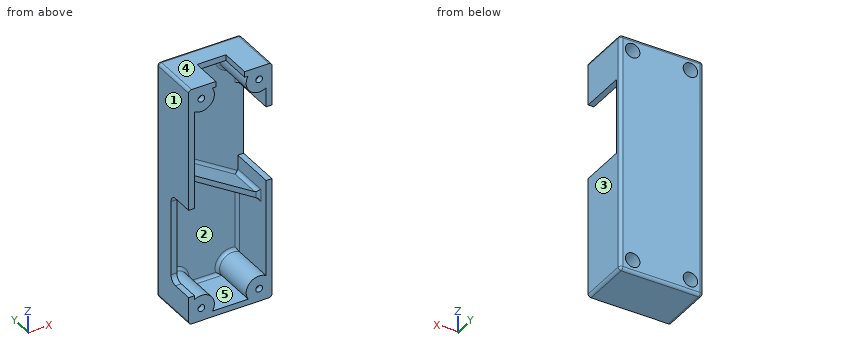
Autodesk Inventor part; units mm, degrees
ref_plane "YZ Plane" through (0, 0, 0) normal (1, 0, 0) x (0, 1, 0)
ref_plane "XZ Plane" through (0, 0, 0) normal (0, 1, 0) x (-1, 0, 0)
ref_plane "XY Plane" through (0, 0, 0) normal (0, 0, 1) x (1, 0, 0)
sketch "Sketch1" plane through (0, 0, 0) normal (0, 1, 0) x (-1, 0, 0)
  line L0 (-4.1759, -63.8889) -> (-35.6719, -63.8889)
  line L1 (-35.6719, -63.8889) -> (-35.6719, 36.1871)
  line L2 (-35.6719, 36.1871) -> (-4.1759, 36.1871)
  line L3 (-4.1759, 36.1871) -> (-4.1759, -63.8889)
  line L4 (-1.6359, -66.4289) -> (-38.2119, -66.4289)
  line L5 (-38.2119, -66.4289) -> (-38.2119, 38.7271)
  line L6 (-38.2119, 38.7271) -> (-1.6359, 38.7271)
  line L7 (-1.6359, 38.7271) -> (-1.6359, -66.4289)
  point P0 (0, 0)
  dimension "d0" = 100.076
  dimension "d1" = 31.496
  dimension "d2" = 2.54
  dimension "d3" = 2.54
  dimension "d4" = 2.54
  dimension "d5" = 2.54
extrude "Extrusion1" add sketch "Sketch1" along normal blind 22.86 contours L0 L1 L2 L3 | L4 L5 L6 L7
extrude "Extrusion2" cut sketch "Sketch1" along normal blind 20.32 contours L0 L1 L2 L3
sketch "Sketch2" plane through (0, 0, 0) normal (0, -1, 0) x (1, 0, 0)
  line L0 (35.6719, 36.1871) -> (35.6719, -63.8889)
  line L1 (38.2119, 38.7271) -> (38.2119, -66.4289)
  line L2 (38.2119, 19.6771) -> (35.6719, 19.6771)
  line L3 (38.2119, -13.3429) -> (35.6719, -13.3429)
  line L4 (4.1759, 36.1871) -> (35.6719, 36.1871)
  point P0 (0, 0)
  point P1 (36.9419, 19.6771)
  point P2 (36.9419, -13.3429)
  dimension "d10" = 16.51
  dimension "d11" = 33.02
extrude "Extrusion3" cut sketch "Sketch2" against normal blind 20.32
sketch "Sketch3" plane through (1.6359, 0, 38.7271) normal (0, 0, 1) x (1, 0, 0)
  line L0 (11.938, 0) -> (24.638, 0)
  line L1 (24.638, 0) -> (24.638, 13.5128)
  line L2 (24.638, 13.5128) -> (11.938, 13.5128)
  line L3 (11.938, 13.5128) -> (11.938, 0)
  line L4 (0, 0) -> (0, 22.86)
  line L5 (36.576, 0) -> (36.576, 22.86)
  line L6 (36.576, 22.86) -> (0, 22.86)
  line L7 (18.288, 22.86) -> (18.288, 0)
  point P0 (-1.6359, 0)
  dimension "d16" = 13.5128
  dimension "d17" = 12.7
  dimension "d18" = 12.7
extrude "Extrusion4" cut sketch "Sketch3" against normal blind 2.54
sketch "Sketch4" plane through (1.6359, 0, -66.4289) normal (-1, 0, 0) x (0, 0, 1)
  line L0 (12.192, 0) -> (51.3334, 0)
  line L1 (51.3334, 0) -> (51.3334, 12.7)
  line L2 (51.3334, 12.7) -> (12.192, 12.7)
  line L3 (12.192, 12.7) -> (12.192, 0)
  line L4 (0, 0) -> (0, 22.86)
  point P0 (66.4289, 0)
  point P1 (31.7627, 0)
  dimension "d21" = 12.192
  dimension "d22" = 12.7
  dimension "d23" = 39.1414
extrude "Extrusion5" cut sketch "Sketch4" against normal blind 2.54
sketch "Sketch5" plane through (0, 22.86, 0) normal (0, 1, 0) x (1, 0, 0)
  circle A0 centre (32.6239, -33.1391) radius 1.4732
  line L0 (38.2119, -38.7271) -> (38.2119, 66.4289)
  line L1 (1.6359, -38.7271) -> (38.2119, -38.7271)
  line L2 (1.6359, 66.4289) -> (1.6359, -38.7271)
  line L3 (1.6359, 13.8509) -> (38.2119, 13.8509)
  line L4 (19.9239, 66.4289) -> (19.9239, -38.7271)
  circle A1 centre (7.2239, -33.1391) radius 1.4732
  circle A2 centre (32.6239, 60.8409) radius 1.4732
  circle A3 centre (7.2239, 60.8409) radius 1.4732
  circle A4 centre (32.6239, -33.1391) radius 3.175
  line L5 (38.2119, -31.941) -> (38.2119, -34.3372)
  line L6 (31.4257, -38.7271) -> (33.822, -38.7271)
  arc A5 (38.2119, -31.941) -> (31.4257, -38.7271) centre (32.6239, -33.1391) ccw
  line L7 (38.2119, -34.3372) -> (38.2119, -38.7271)
  line L8 (38.2119, -38.7271) -> (33.822, -38.7271)
  line L9 (38.2119, -38.7271) -> (1.6359, -38.7271)
  circle A6 centre (7.2239, -33.1391) radius 3.175
  line L10 (1.6359, -31.941) -> (1.6359, -34.3372)
  arc A7 (8.422, -38.7271) -> (1.6359, -31.941) centre (7.2239, -33.1391) ccw
  line L11 (1.6359, -34.3372) -> (1.6359, -38.7271)
  line L12 (38.2119, 66.4289) -> (38.2119, -38.7271)
  line L13 (1.6359, -38.7271) -> (1.6359, 66.4289)
  circle A8 centre (32.6239, 60.8409) radius 3.175
  arc A9 (31.4257, 66.4289) -> (38.2119, 59.6428) centre (32.6239, 60.8409) ccw
  circle A10 centre (7.2239, 60.8409) radius 3.175
  arc A11 (1.6359, 59.6428) -> (8.422, 66.4289) centre (7.2239, 60.8409) ccw
  line L14 (38.2119, 66.4289) -> (1.6359, 66.4289)
  point P0 (0, 0)
  point P1 (1.6359, 59.6428)
  point P2 (38.2119, 59.6428)
  point P3 (8.422, -38.7271)
  point P4 (1.6359, -31.941)
  dimension "d27" = 2.9464
  dimension "d28" = 5.588
  dimension "d29" = 5.588
  dimension "d30" = 6.35
extrude "Extrusion6" add sketch "Sketch5" against normal up to surface (22.86 mm away) contours A0 | L1 A5 L0 | A9 L14 L0 | L1 L2 A7 | L2 L14 A11 | A1 | A2 | A3 | A4 | A6 | A8 | A10
extrude "Extrusion7" cut sketch "Sketch5" against normal blind 20.32 contours A0 | A1 | A2 | A3 | A4 | A6 | A8 | A10
extrude "Extrusion8" cut sketch "Sketch5" against normal blind 22.86 contours A0 | A1 | A2 | A3
fillet "Fillet2" radius 3.175 2 edges at (2.9059, 12.7, -54.2369) (2.9059, 12.7, -15.0955)
fillet "Fillet3" radius 1.27 8 edges at (38.2119, 22.86, -13.8509) (38.2119, 11.43, 38.7271) (19.9239, 22.86, 38.7271) (1.6359, 22.86, -13.8509) (38.2119, 11.43, -66.4289) (19.9239, 22.86, -66.4289) (1.6359, 11.43, 38.7271) (1.6359, 11.43, -66.4289)
sketch "Sketch8" plane through (0, 0, 0) normal (0, -1, 0) x (1, 0, 0)
  line L0 (1.6359, -15.0955) -> (4.1759, -15.0955)
  line L1 (4.1759, -15.0955) -> (17.1299, -15.0955)
  line L2 (17.1299, -15.0955) -> (17.1299, -54.5295)
  line L3 (17.1299, -54.5295) -> (4.1759, -54.5295)
  line L4 (4.1759, -54.5295) -> (4.1759, -15.0955)
  line L5 (35.6719, -13.3429) -> (35.6719, -56.0065)
  line L6 (35.6719, -13.3429) -> (24.7499, -13.3429)
  line L7 (24.7499, -13.3429) -> (24.7499, 19.5815)
  line L8 (24.7499, 19.5815) -> (35.6719, 19.5815)
  line L9 (35.6719, 19.5815) -> (35.6719, -13.3429)
  line L10 (4.1759, -4.9355) -> (35.6719, -24.2565)
  line L11 (4.1759, -4.9355) -> (4.1759, -2.3955)
  line L12 (2.9059, 37.4571) -> (2.9059, -65.1589)
  line L13 (35.6719, -24.2565) -> (35.6719, -21.7165)
  line L14 (4.1759, -2.3955) -> (35.6719, -21.7165)
  point P0 (0, 0)
  point P1 (24.7499, 3.1193)
  dimension "d44" = 10.922
  dimension "d45" = 12.954
  dimension "d46" = 2.54
  dimension "d47" = 2.54
  dimension "d48" = 31.75
  dimension "d49" = 10.16
extrude "Extrusion11" add sketch "Sketch8" against normal blind 20.32 contours L5 L10 L11 L14
extrude "Extrusion12" cut sketch "Sketch8" against normal blind 5.08 contours L5 L10 L11 L14
fillet "Fillet4" radius 1.27 18 edges at (4.1759, 12.7, -2.3955) (4.1759, 20.32, 12.9546) (19.9239, 20.32, -12.056) (4.1759, 5.08, -3.6655) (19.9239, 20.32, -14.596) (35.6719, 12.7, -24.2565) (35.6719, 5.08, -22.9865) (35.6719, 20.32, -40.1315) (35.6719, 20.32, 23.9909) (28.5827, 20.32, 29.098) (19.9239, 20.32, 36.1871) (19.9239, 20.32, -63.8889) (28.5827, 20.32, -56.7998) (11.265, 20.32, -56.7998) (4.1759, 20.32, -30.471) (11.265, 20.32, 29.098) (4.1759, 12.7, -4.9355) (35.6719, 12.7, -21.7165)
properties part number "CaseTop"
Could you check a few things on this model? Use its own coordinates, in mm. Face numbers are marked on the shaded views. A direction names the side the tool comes from. Coordinates: 2 decimals unless noted, no trailing zeros. Order: outer loops, then holes, each group sorted by start corner. A loop starts at its lowest first (then second) coordinate and runs counter-clockwise, first axis right, second up. Notation, with made-up numbers: (84.5, 28) -> (118.5, 28) arc R7 cw to (118.5, 35) -> close; hole circle Ø8 at (-12, 35.25). An arc over 180 degrees is marked (long way). One line per item, written item: value. Start each with the question number.
1) We'd pull the mould along X, two halves only. Please class the marked faces 3, 4 and 5: +X half, -X half, draft (parallel to the pull), parting line (faces both ways), or undercut.
2) If I drill on L1, parallel to X at y = 13.25, z = -25.5; L2, parallel to Z at x = 27.5, y = 4.75; L3, parallel to Z at x = 15.5, y = 18.25, over which ranges is the centre line in solid material (lowest first)? Write a range as [from, to].
3) I'm going to push flat-ended pins straight in: pin 1 (1 mm diameter, centred on x = 15.5, y = 4, fed in from +Z); pin 2 (0.8 mm diameter, centred on x = 22, z = 37, fed in from -Y); pin 3 (3 mm diameter, centred on x = 2.5, z = -33.5, fed in from -Y); pin 4 (2.5 mm diameter, centred on x = 32.62, z = -60.84, fed in from -Y). Where does each tip first touch, or does it pass through?
4) Which directions (+Z, -Z, +X, -X, +Y, -Y) give clear straight access to the entire face, cutting with the end or side of a thin tool? Please do the marked faces 1 and 2.
5) Imagine slicing it at B-B on y = 15.75. Count the separate pieces of the cut face and the enclosed holes in it, plus the area to 3 significant figures.
6) Imagine slicing it at A-A on z = -30. List the corners of the cut face in (x, y) for me.
Answer list:
1. face 3: +X half
1. face 4: draft
1. face 5: undercut
2. L1: x = [1.64, 4.18], [35.67, 38.21]
2. L2: z = [-66.43, -63.89], [-63.37, -58.31], [30.61, 35.67], [36.19, 38.73]
2. L3: z = [-66.43, -63.89], [-11.88, -9.34], [36.19, 38.73]
3. pin 1: stops at z = -63.89
3. pin 2: stops at y = 13.51
3. pin 3: stops at y = 12.7
3. pin 4: passes through
4. face 1: +Z, -Z, -X, +Y, -Y
4. face 2: -Y
5. separate pieces: 1
5. enclosed holes: 5
5. area: 837 mm2
6. outline: (1.64, 12.7) -> (4.18, 12.7) -> (4.18, 19.05) arc R1.27 cw to (5.45, 20.32) -> (34.4, 20.32) arc R1.27 cw to (35.67, 19.05) -> (35.67, 0) -> (38.21, 0) -> (38.21, 21.59) arc R1.27 ccw to (36.94, 22.86) -> (2.91, 22.86) arc R1.27 ccw to (1.64, 21.59) -> close
